Verification items for this drawing (mm, ordinates from the low corner). A direction names the side the tool comes from. Coordinates: 2 decimals unless noted, no trailing zeros. Order: outer loops, then holes, each group sorted by start corner. A loop starts at its lowest first (then second) coordinate and runs counter-clockwise, first axis right, second up. Notation, with made-up numbers: (49.5, -36.75) -> (99.5, -36.75) arc R21 ccw to (99.5, -8.75) -> close; hole circle Ø5 at (37, 77.5). An arc over 180 degrees is marked (long way). Write item = value, one per line. Start each with the question number.
1. Set-up check for the marked faces 5, 6, 7 and 8: record each of +Z, -Z, +X, -X, +Y, -Y from which the full face is reachable in a straight line by a thin tool's end or side.
2. Cross-section at C-C on x = 92.5. Record the cut outline in (y, z).
3. Go/stop test with a flat-tipped pin: P1, Ø12, axis at x = 117.5, z = 14, coming from the +Y side. Record where the tip stops, or that it passes through.
4. Cross-section at B-B on z = 14. Record the cut outline in (x, y), plus the area to 3 significant figures.
5. Cross-section at D-D on y = 117. Record the cut outline in (x, z).
6. Release check for a two-part mould opening along X. For the marked faces 1, 2, 3 and 4 record: +X half, -X half, draft (parallel to the pull), parting line (faces both ways), or undercut.
7. Cross-section at A-A on y = 63.5. Record the cut outline in (x, z), plus the area to 3 significant figures.
8. Thickness scan on line 1 along X through (y, z) = (78, 11); line 2 along Y through (x, z) = (183, 20.5); line 3 along X through (y, z) = (37, 6.25). Record the ranges inside material, lowest first. Write a range as from..to.
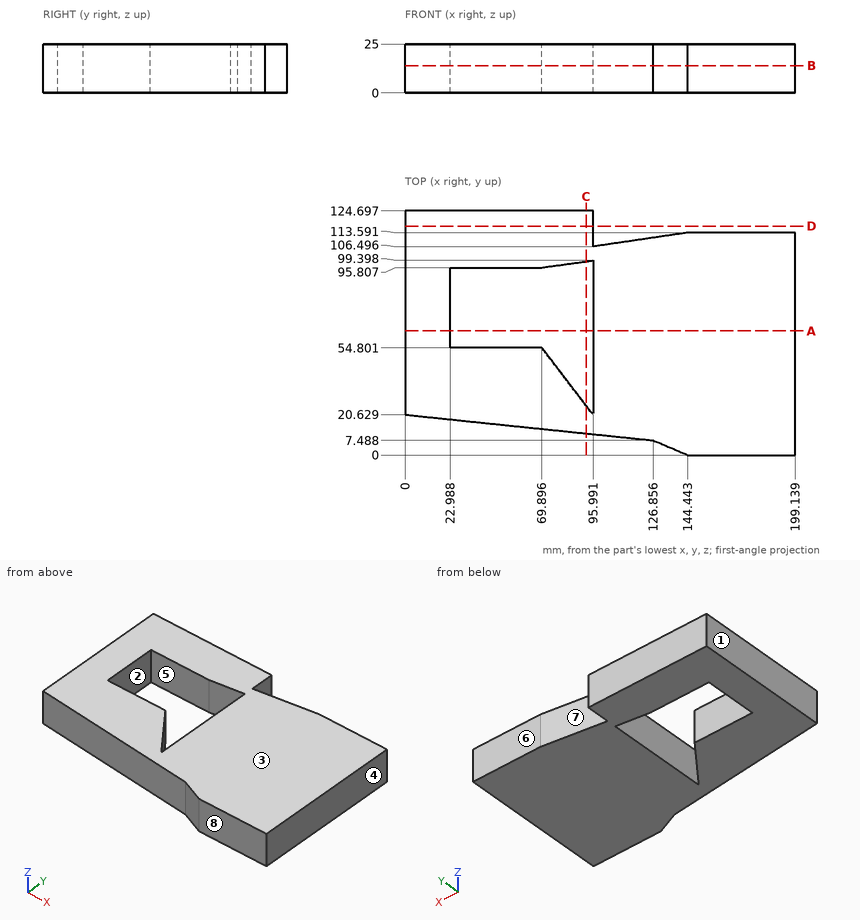
Worked out:
q1.face_5 = +Z, -Z
q1.face_6 = +Z, -Z, +X, +Y
q1.face_7 = +Z, -Z, +Y
q1.face_8 = +Z, -Z, +X, -X, -Y
q2.outline = (11.05, 0) -> (25.2, 0) -> (25.2, 25) -> (11.05, 25) -> close; (98.92, 0) -> (124.7, 0) -> (124.7, 25) -> (98.92, 25) -> close
q3.P1 = 110.52
q4.outline = (0, 20.63) -> (126.86, 7.49) -> (144.44, 0) -> (199.14, 0) -> (199.14, 113.59) -> (144.44, 113.59) -> (95.99, 106.5) -> (95.99, 124.7) -> (0, 124.7) -> close; hole (22.99, 54.8) -> (69.9, 54.8) -> (95.99, 20.63) -> (95.99, 99.4) -> (69.9, 95.81) -> (22.99, 95.81) -> close
q4.area = 18,200 mm²
q5.outline = (0, 0) -> (95.99, 0) -> (95.99, 25) -> (0, 25) -> close
q6.face_1 = -X half
q6.face_2 = undercut
q6.face_3 = draft
q6.face_4 = +X half
q7.outline = (0, 0) -> (22.99, 0) -> (22.99, 25) -> (0, 25) -> close; (95.99, 0) -> (199.14, 0) -> (199.14, 25) -> (95.99, 25) -> close
q7.area = 3,150 mm²
q8.line_1 = 0..22.99, 95.99..199.14
q8.line_2 = 0..113.59
q8.line_3 = 0..83.49, 95.99..199.14
